Can you work these out from the model? Positions are in its coordinate system, mm. Face numbers are marked on the shaded views. Give positions to 0.01 mm unless a question says otherwise; leave off trailing zeros. Loops run counter-clockwise (first coordinate to the right, second up) from the corner with the lowest first, then second, coordinate; pieces in that order, holes last. Notation, with made-up numbers: (11.25, 65.25) - (42.25, 65.25) arc R26 ccw to (42.25, 90.25) - close; hole circle Ø2 at (-38, -24.5). An arc over 180 degrees is marked (long way). Write item = value, one per line.
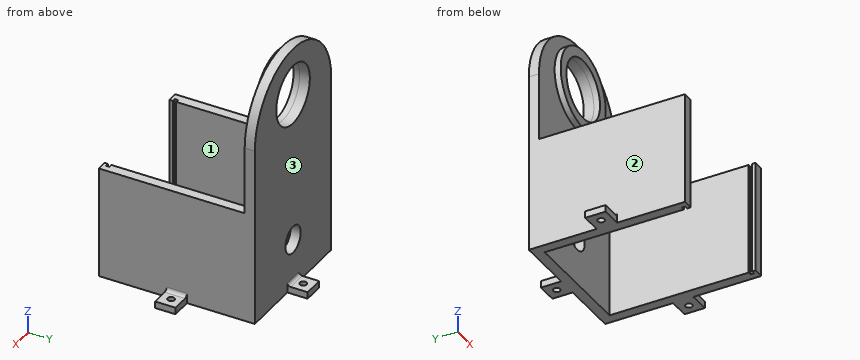
from build123d import *

# Parameters (mm, degrees)
SKETCH1_W           = 50.8
SKETCH1_H           = 58.42
SKETCH1_W_2         = 43.18
SKETCH1_H_2         = 50.8
EXTRUDE_THIN1_DEPTH = 41.91
SKETCH2_R           = 5.08
CUT_EXTRUDE1_DEPTH  = 5.08
SKETCH3_W           = 43.18
SKETCH3_H           = 41.91
CUT_EXTRUDE2_DEPTH  = 5.08
SKETCH4_W           = 7.62
SKETCH4_H           = 7.62
SKETCH4_R           = 1.27
BOSS_EXTRUDE1_DEPTH = 2.54
SKETCH5_W           = 41.91
SKETCH5_H           = 1.27
CUT_EXTRUDE3_DEPTH  = 1.27
SKETCH6_R           = 11.176
BOSS_EXTRUDE2_DEPTH = 3.81
FILLET2_R           = 1.27
SKETCH7_R           = 14.986
SKETCH7_R_2         = 11.176
BOSS_EXTRUDE3_DEPTH = 2.286


with BuildPart() as part:
    # Sketch1 → Extrude-Thin1 (new body)
    with BuildSketch(Plane.XY):
        Rectangle(SKETCH1_W, SKETCH1_H)
        Rectangle(SKETCH1_W_2, SKETCH1_H_2, mode=Mode.SUBTRACT)
    extrude(amount=EXTRUDE_THIN1_DEPTH)

    # Sketch2 → Cut-Extrude1 (cut)
    with BuildSketch(Plane(origin=(0, 29.21, 0), x_dir=(1, 0, 0), z_dir=(0, 1, 0))):
        with Locations(Location((0, -18.415, 0), (0, 0, 180))):
            Circle(SKETCH2_R)
    extrude(amount=-CUT_EXTRUDE1_DEPTH, mode=Mode.SUBTRACT)

    # Sketch3 → Cut-Extrude2 (cut)
    with BuildSketch(Plane.XZ.offset(29.21)):
        with Locations((0, 20.955)):
            Rectangle(SKETCH3_W, SKETCH3_H)
    extrude(amount=-CUT_EXTRUDE2_DEPTH, mode=Mode.SUBTRACT)

    # Sketch4 → Boss-Extrude1 (add)
    # profile 1 of 3: a face of its own
    with BuildSketch(Plane(origin=(0, 0, 0), x_dir=(-1, 0, 0), z_dir=(0, 0, -1))):
        with Locations((29.21, 0)):
            Rectangle(SKETCH4_W, SKETCH4_H)
        with Locations((29.21, 0)):
            Circle(SKETCH4_R, mode=Mode.SUBTRACT)
    # profile 2 of 3: a face of its own
    with BuildSketch(Plane(origin=(0, 0, 0), x_dir=(-1, 0, 0), z_dir=(0, 0, -1))):
        with Locations((-29.21, 0)):
            Rectangle(SKETCH4_W, SKETCH4_H)
        with Locations((-29.21, 0)):
            Circle(SKETCH4_R, mode=Mode.SUBTRACT)
    # profile 3 of 3: a face of its own
    with BuildSketch(Plane(origin=(0, 0, 0), x_dir=(-1, 0, 0), z_dir=(0, 0, -1))):
        with Locations((0, 33.02)):
            Rectangle(SKETCH4_W, SKETCH4_H)
        with Locations((0, 33.02)):
            Circle(SKETCH4_R, mode=Mode.SUBTRACT)
    extrude(amount=-BOSS_EXTRUDE1_DEPTH)

    # Sketch5 → Cut-Extrude3 (cut)
    with BuildSketch(Plane.ZY.offset(-21.59)):
        with Locations((20.955, -27.305)):
            Rectangle(SKETCH5_W, SKETCH5_H)
    cut_extrude3 = extrude(amount=-CUT_EXTRUDE3_DEPTH, mode=Mode.SUBTRACT)

    # Mirror1: Cut-Extrude3 across plane
    add(cut_extrude3.mirror(Plane.ZY), mode=Mode.SUBTRACT)

    # Sketch6 → Boss-Extrude2 (add)
    with BuildSketch(Plane(origin=(0, 29.21, 0), x_dir=(1, 0, 0), z_dir=(0, 1, 0))):
        with BuildLine():
            Line((25.4, -67.31), (25.4, -41.91))
            Line((25.4, -41.91), (-25.4, -41.91))
            Line((-25.4, -41.91), (-25.4, -67.31))
            ThreePointArc((-25.4, -67.31), (0, -92.71), (25.4, -67.31))
        make_face()
        with Locations(Location((0, -74.93, 0), (0, 0, 180))):
            Circle(SKETCH6_R, mode=Mode.SUBTRACT)
    extrude(amount=-BOSS_EXTRUDE2_DEPTH)

    # Fillet2
    fillet2_edges = [part.edges().sort_by_distance(p)[0] for p in [
        (-25.4, 0, 2.54),
        (25.4, 0, 2.54),
        (0, 29.21, 2.54),
    ]]
    fillet(fillet2_edges, radius=FILLET2_R)

    # Sketch7 → Boss-Extrude3 (add)
    with BuildSketch(Plane.XZ.offset(-25.4)):
        with Locations((0, 74.93)):
            Circle(SKETCH7_R)
        with Locations(Location((0, 74.93, 0), (0, 0, 180))):
            Circle(SKETCH7_R_2, mode=Mode.SUBTRACT)
    extrude(amount=BOSS_EXTRUDE3_DEPTH)


solid = part.part
Q1. Imagine slicing it at D-D, the plane y = 0. Write out the boundary of the cut face in (x, z), then the cut area to 3 significant figures.
Output:
outline = (-33.02, 0) - (-30.48, 0) - (-30.48, 2.54) - (-33.02, 2.54) - close; (-27.94, 0) - (-21.59, 0) - (-21.59, 41.91) - (-25.4, 41.91) - (-25.4, 3.81) arc R1.27 cw to (-26.67, 2.54) - (-27.94, 2.54) - close; (21.59, 0) - (27.94, 0) - (27.94, 2.54) - (26.67, 2.54) arc R1.27 cw to (25.4, 3.81) - (25.4, 41.91) - (21.59, 41.91) - close; (30.48, 0) - (33.02, 0) - (33.02, 2.54) - (30.48, 2.54) - close
area = 346 mm2
Q2. Imagine slicing it at B-B, the plane y = -21. Write out the boundary of the cut face in (x, z).
Output:
outline = (-25.4, 0) - (-21.59, 0) - (-21.59, 41.91) - (-25.4, 41.91) - close; (21.59, 0) - (25.4, 0) - (25.4, 41.91) - (21.59, 41.91) - close
Q3. For pin 1 (1.9 mm diameter, centred on y = 33, z = 2, fed in from +X); pin 2 (1.1 mm diameter, centred on x = -30.5, z = 2, fed in from -Y); pin 3 (5 mm diameter, centred on x = 19.5, y = 9, fed in from +Z); pin 4 (1.5 mm diameter, centred on x = -29.21, y = 0, fed in from -Z), each with a flat end and sliding along its axis, tell me the tip position at first contact or that it passes through.
Output:
pin_1 = 3.81
pin_2 = -3.81
pin_3 = 41.91
pin_4 = through
Q4. We'd pull the mould along X, two halves only. Please class the marked faces 1, 2 and 3: released by +X, released by -X, zero draft, split by the parting line, or undercut.
Output:
face_1 = undercut
face_2 = released by -X
face_3 = zero draft
Q5. Imagine slicing it at A-A, the plane x = 29.21. Write out the boundary of the cut face in (y, z), then the cut area to 3 significant figures.
Output:
outline = (-3.81, 0) - (-1.27, 0) - (-1.27, 2.54) - (-3.81, 2.54) - close; (1.27, 0) - (3.81, 0) - (3.81, 2.54) - (1.27, 2.54) - close
area = 12.9 mm2
Q6. I need wall thicknesses on L1, parallel to Z at x = 0, y = 26.6 (3 decimals); L2, parallel to X at y = -2.5, z = 33; L3, parallel to Y at x = 29.21, z = 1.45. Which ranges of each line are inside material? Lowest first, please.
Output:
L1 = 0 to 13.335, 23.495 to 63.754, 86.106 to 92.71
L2 = -25.4 to -21.59, 21.59 to 25.4
L3 = -3.81 to -1.27, 1.27 to 3.81
Q7. Imagine slicing it at C-C, the plane x = 0. Write out the boundary of the cut face in (y, z) (3 decimals).
Output:
outline = (23.114, 59.944) - (25.4, 59.944) - (25.4, 23.495) - (29.21, 23.495) - (29.21, 63.754) - (23.114, 63.754) - close; (23.114, 86.106) - (29.21, 86.106) - (29.21, 92.71) - (25.4, 92.71) - (25.4, 89.916) - (23.114, 89.916) - close; (25.4, 0) - (31.75, 0) - (31.75, 2.54) - (30.48, 2.54) arc R1.27 cw to (29.21, 3.81) - (29.21, 13.335) - (25.4, 13.335) - close; (34.29, 0) - (36.83, 0) - (36.83, 2.54) - (34.29, 2.54) - close
